from build123d import *

# Parameters (mm, degrees)
F0_W     = 95
F0_H     = 25
F0_R     = 2.75
F0_R_2   = 3.25
F0_R_3   = 4
F1_DEPTH = 8
F2_D     = 8
F3_SIZE  = 3


with BuildPart() as f1:
    # F0 (on Front) → F1 (new body)
    with BuildSketch(Plane.XZ):
        with Locations((47.5, 12.5)):
            Rectangle(F0_W, F0_H)
        with Locations((6.5, 5)):
            Circle(F0_R, mode=Mode.SUBTRACT)
        with Locations((88.5, 5)):
            Circle(F0_R, mode=Mode.SUBTRACT)
        with Locations((18.5, 17.5)):
            Circle(F0_R_2, mode=Mode.SUBTRACT)
        with Locations((6.5, 20)):
            Circle(F0_R, mode=Mode.SUBTRACT)
        with Locations((47.5, 12.5)):
            Circle(F0_R_3, mode=Mode.SUBTRACT)
        with Locations((76.5, 17.5)):
            Circle(F0_R_2, mode=Mode.SUBTRACT)
        with Locations((88.5, 20)):
            Circle(F0_R, mode=Mode.SUBTRACT)
        with Locations((47.5, 12.5)):
            Circle(F0_R_3)
    extrude(amount=F1_DEPTH)

    # F2 (through all)
    with Locations(Plane(origin=(0, 0, 0), x_dir=(1, 0, 0), z_dir=(0, 1, 0))):
        with Locations((47.5, -12.5)):
            Hole(F2_D / 2)

    # F3
    f3_edges = [f1.edges().sort_by_distance(p)[0] for p in [
        (95, -4, 25),
        (95, -4, 0),
        (0, -4, 25),
        (0, -4, 0),
    ]]
    chamfer(f3_edges, length=F3_SIZE)


solid = f1.part
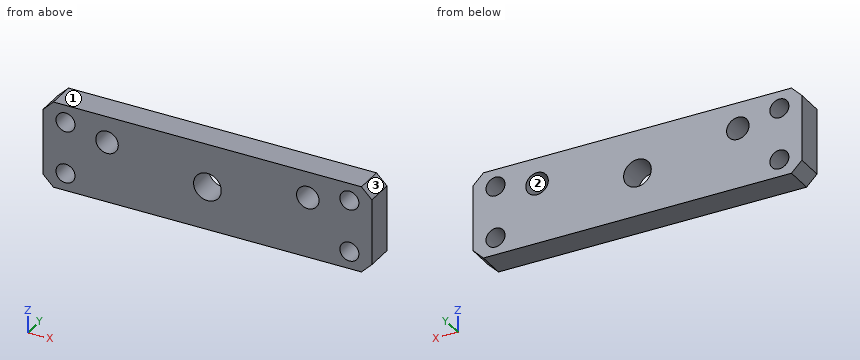
The listing builds one solid part. Answer for the finished solid, in the listing's coordinates (mm). Face numbers are marked on the shaded views. Give positions to 0.01 mm unless a question says otherwise; leave off trailing zeros. Loops run counter-clockwise (first coordinate to the right, second up) from the corner with the lowest first, then second, coordinate; pieces in that order, holes last.
Item 1: Determine the mould class of the marked faces 1, 2 and 3 for opening direction X: +X half, -X half, draft (parallel to the pull), parting line (faces both ways), or undercut.
Derived:
face 1: draft
face 2: undercut
face 3: +X half
Item 2: A cutting plane is placed at C-C (y = -1.5). Give the vertices of the cut face in (x, z), then the cut area to 3 significant figures.
Derived:
outline: (0, 3) - (3, 0) - (92, 0) - (95, 3) - (95, 22) - (92, 25) - (3, 25) - (0, 22) - close; hole circle Ø5.5 at (6.5, 5); hole circle Ø5.5 at (6.5, 20); hole circle Ø6.5 at (18.5, 17.5); hole circle Ø8 at (47.5, 12.5); hole circle Ø6.5 at (76.5, 17.5); hole circle Ø5.5 at (88.5, 5); hole circle Ø5.5 at (88.5, 20)
area: 2,150 mm2
Item 3: A cutting plane is placed at A-A (z = 5). Give the vertices of the cut face in (x, y), then the cut area to 3 significant figures.
Derived:
outline: (0, -8) - (3.75, -8) - (3.75, 0) - (0, 0) - close; (9.25, -8) - (85.75, -8) - (85.75, 0) - (9.25, 0) - close; (91.25, -8) - (95, -8) - (95, 0) - (91.25, 0) - close
area: 672 mm2
Item 4: A cutting plane is placed at D-D (x = 6.5). Give the vertices of the cut face in (y, z), then the cut area to 3 significant figures.
Derived:
outline: (-8, 0) - (0, 0) - (0, 2.25) - (-8, 2.25) - close; (-8, 7.75) - (0, 7.75) - (0, 17.25) - (-8, 17.25) - close; (-8, 22.75) - (0, 22.75) - (0, 25) - (-8, 25) - close
area: 112 mm2
Item 5: This flat-tipped pin is pushed along its axis until it touches: pin 1 Ø5 at (x, z) = (88.5, 5) entering from -Y. Where does it stop, or does it pass through?
Derived:
pin 1: passes through
Item 6: A cutting plane is placed at B-B (x = 76.5). Give the vertices of the cut face in (y, z).
Derived:
outline: (-8, 0) - (0, 0) - (0, 14.25) - (-8, 14.25) - close; (-8, 20.75) - (0, 20.75) - (0, 25) - (-8, 25) - close
Item 7: Find the intervals of material crossed by line 1 along Z through (x, y) = (88.5, -6); line 2 along Z through (x, y) = (76.5, -4); line 3 along Z through (x, y) = (47.5, -3.75), in increasing order.
Derived:
line 1: z = 0 to 2.25, 7.75 to 17.25, 22.75 to 25
line 2: z = 0 to 14.25, 20.75 to 25
line 3: z = 0 to 8.5, 16.5 to 25
